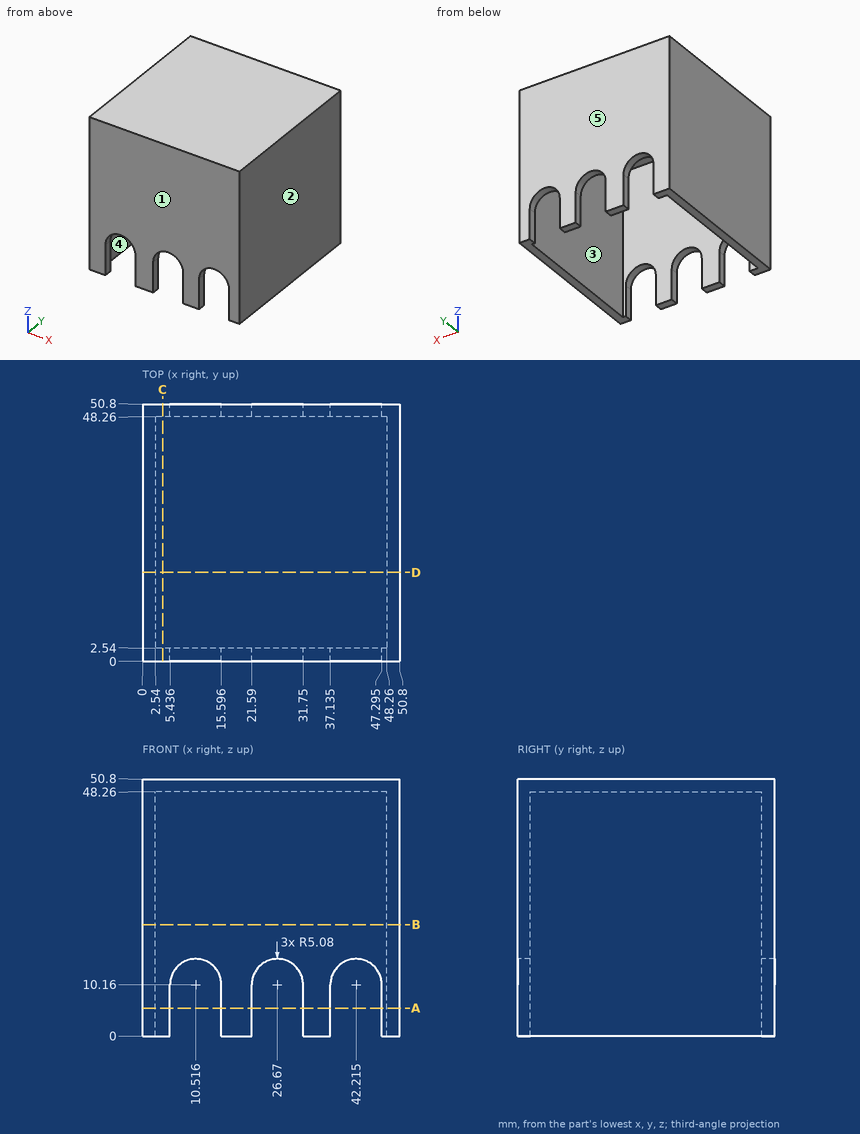
Drawing for the job (mm, zero at the part's lowest x, y, z). A direction names the side the tool comes from. Give positions to 0.01 mm unless a question says otherwise; leave off trailing zeros. Loops run counter-clockwise (first coordinate to the right, second up) from the corner with the lowest first, then second, coordinate; pieces in that order, holes last.
1) Drop a flat-ended pin along its axis: P1, Ø13.5, axis at x = 34.5, y = 16, coming from the -Z side. Give the stop position or say it passes through.
Values follow:
P1: stops at z = 48.26
2) Band-saw the part on C-C on x = 4. List the corners of the cut face in (y, z).
Values follow:
outline: (0, 0) - (2.54, 0) - (2.54, 48.26) - (48.26, 48.26) - (48.26, 0) - (50.8, 0) - (50.8, 50.8) - (0, 50.8) - close
3) Two-plate mould, pull along Y, no slides. Class the marked faces 1, 2 and 3: released by +Y, released by -Y, zero draft, split by the parting line, or undercut.
Values follow:
face 1: released by -Y
face 2: zero draft
face 3: undercut
4) Band-saw the part on A-A on z = 5.5. State how many separate pieces and enclosed holes the cut face has.
Values follow:
separate pieces: 6
enclosed holes: 0
5) 3-axis set-ups, long thin cutter, end or side, ignore diameter. For the marked faces 4 and 5: which of +Z, -Z, +X, -X, +Y, -Y reach the whole face in a straight line?
Values follow:
face 4: -Z
face 5: +Z, -Z, +X, -X, +Y
6) Band-saw the part on B-B on z = 22. List the corners of the cut face in (x, y).
Values follow:
outline: (0, 0) - (50.8, 0) - (50.8, 50.8) - (0, 50.8) - close; hole (2.54, 2.54) - (48.26, 2.54) - (48.26, 48.26) - (2.54, 48.26) - close
7) Probe line 1 along Y through (x, z) = (4, 32); line 2 along Z through (x, y) = (47.5, 47). List the from-to ranges inside material, lowest first.
Values follow:
line 1: y = 0 to 2.54, 48.26 to 50.8
line 2: z = 48.26 to 50.8
